from build123d import *

# Parameters (mm, degrees)
F1_W     = 43.941932
F1_H     = 35.796363
F2_DEPTH = 25.4
F0_W     = 74.497212
F0_H     = 43.208381
F3_DEPTH = 25.4
F4_R     = 5.08
F5_R     = 5.08


with BuildPart() as f2:
    # F1 (on Right) → F2 (new body)
    with BuildSketch(Plane.YZ):
        with Locations((5.488838, -17.898181)):
            Rectangle(F1_W, F1_H)
    extrude(amount=F2_DEPTH)

    # F0 (on Top) → F3 (join)
    with BuildSketch(Plane.XY):
        with Locations((11.949877, 5.810783)):
            Rectangle(F0_W, F0_H)
    extrude(amount=F3_DEPTH)

    # F4
    f4_edges = [f2.edges().sort_by_distance(p)[0] for p in [
        (49.198483, 5.810783, 0),
    ]]
    fillet(f4_edges, radius=F4_R)

    # F5
    f5_edges = [f2.edges().sort_by_distance(p)[0] for p in [
        (-25.298729, 5.810783, 0),
    ]]
    fillet(f5_edges, radius=F5_R)


solid = f2.part
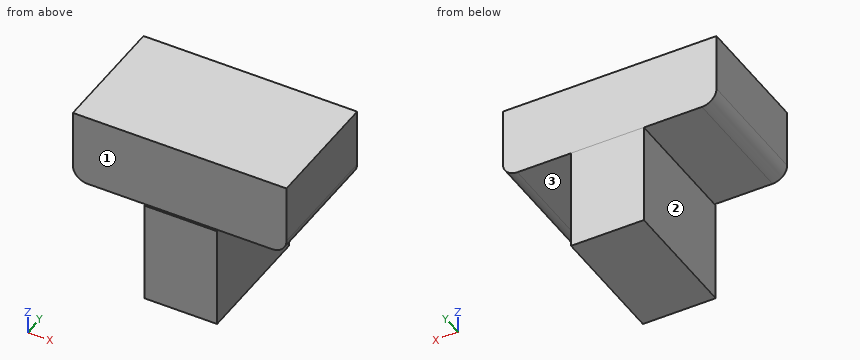
The listing builds one solid part. Answer for the finished solid, in the listing's coordinates (mm). Face numbers are marked on the shaded views. A direction names the side the tool comes from. Round coordinates to 2 decimals unless told otherwise and drop trailing zeros. Order: outer loops, then holes, each group sorted by start corner. A loop starts at its lowest first (then second) coordinate and runs counter-clockwise, first axis right, second up. Notation, with made-up numbers: (37, -1) - (93, -1) arc R18 cw to (93, 7) - close; hole circle Ø8 at (74, 41). An arc over 180 degrees is marked (long way). Write item = value, one per line. Start each with the question number.
1) Section B-B, the plane z = 20 is taken. Write down the section's boundary in (x, y), plus the area to 3 significant figures.
2) Section A-A, the plane y = 13.5 is taken. Write down the section's boundary in (x, z), plus the area to 3 significant figures.
3) Straight lines are drawn through the part: L1, parallel to X at y = 1, z = -13.5; L2, parallel to Y at x = 31, z = 13. For each, find the intervals that lie inside material, in ascending order.
4) Given pin 1 (3 mm diameter, centred on y = 8.5, z = 1, fed in from -X); pin 2 (1 mm diameter, centred on x = 33, y = 10, fed in from -Z); pin 3 (5 mm diameter, centred on y = -1, z = -15.5, fed in from -X), each flat-ended and moving along its own axis, determine where each tip first touches the part or whether it passes through.
5) For the marked faces 1, 2 and 3, determine the directions among +Z, -Z, +X, -X, +Y, -Y from which every point of the face is accessible in a straight line to the end or side of a thin tool.
6) Section C-C, the plane x = 29 is taken. Write down the section's boundary in (y, z), plus the area to 3 significant figures.
Results list:
q1.outline = (-25.3, -15.79) - (49.2, -15.79) - (49.2, 27.41) - (-25.3, 27.41) - close
q1.area = 3,220 mm^2
q2.outline = (-25.3, 5.08) arc R5.08 ccw to (-20.22, 0) - (0, 0) - (0, -35.8) - (25.4, -35.8) - (25.4, 0) - (44.12, 0) arc R5.08 ccw to (49.2, 5.08) - (49.2, 25.4) - (-25.3, 25.4) - close
q2.area = 2,790 mm^2
q3.L1 = 0 to 25.4
q3.L2 = -15.79 to 27.41
q4.pin_1 = -24.59
q4.pin_2 = 0
q4.pin_3 = 0
q5.face_1 = +Z, +X, -X, -Y
q5.face_2 = -Z, -X, +Y, -Y
q5.face_3 = -Z, +X, +Y, -Y
q6.outline = (-15.79, 0) - (27.41, 0) - (27.41, 25.4) - (-15.79, 25.4) - close
q6.area = 1,100 mm^2
